```python
from build123d import *

# Parameters (mm, degrees)
SKETCH1_W           = 57.15
SKETCH1_H           = 57.15
BOSS_EXTRUDE1_DEPTH = 9.525
SKETCH5_R           = 12.281683601
SKETCH5_R_2         = 3.302
CUT_EXTRUDE1_DEPTH  = 3.175
SKETCH7_W           = 57.15
SKETCH7_H           = 57.15
CUT_EXTRUDE2_DEPTH  = 9.652
SKETCH10_R          = 3.175
CUT_EXTRUDE4_DEPTH  = 79.640756641


with BuildPart() as part:
    # Sketch1 → Boss-Extrude1 (new body)
    with BuildSketch(Plane(origin=(0, 0, 0), x_dir=(1, 0, 0), z_dir=(0, 1, 0))):
        with Locations((28.575, -28.575)):
            Rectangle(SKETCH1_W, SKETCH1_H)
    extrude(amount=BOSS_EXTRUDE1_DEPTH)

    # Sketch5 → Cut-Extrude1 (cut)
    # profile 1 of 5: a face of its own
    with BuildSketch(Plane(origin=(0, 9.525, 0), x_dir=(1, 0, 0), z_dir=(0, 1, 0))):
        with BuildLine():
            ThreePointArc((32.232759975, -45.931274041), (32.269707879, -38.244901062), (36.493054182, -31.822670864))
            ThreePointArc((36.493054182, -31.822670864), (28.575, -34.715841801), (20.656945818, -31.822670864))
            ThreePointArc((20.656945818, -31.822670864), (24.880292121, -38.244901062), (24.917240025, -45.931274041))
            ThreePointArc((24.917240025, -45.931274041), (28.575, -50.807525402), (32.232759975, -45.931274041))
        make_face()
    # profile 2 of 5: a face of its own
    with BuildSketch(Plane(origin=(0, 9.525, 0), x_dir=(1, 0, 0), z_dir=(0, 1, 0))):
        with Locations((28.575, -22.434158199)):
            Circle(SKETCH5_R)
        with Locations((28.575, -22.434158199)):
            Circle(SKETCH5_R_2, mode=Mode.SUBTRACT)
    # profile 3 of 5: a face of its own
    with BuildSketch(Plane(origin=(0, 9.525, 0), x_dir=(1, 0, 0), z_dir=(0, 1, 0))):
        with Locations((28.575, -22.434158199)):
            Circle(SKETCH5_R_2)
    # profile 4 of 5: a face of its own
    with BuildSketch(Plane(origin=(0, 9.525, 0), x_dir=(1, 0, 0), z_dir=(0, 1, 0))):
        with BuildLine():
            ThreePointArc((16.485282438, -24.597137937), (17.93875, -16.293316399), (24.403336619, -10.882665797))
            ThreePointArc((24.403336619, -10.882665797), (16.729848967, -11.329075886), (10.054780753, -7.517887219))
            ThreePointArc((10.054780753, -7.517887219), (4.002943212, -8.247474598), (6.397020778, -13.853313338))
            ThreePointArc((6.397020778, -13.853313338), (13.035141089, -17.72849765), (16.485282438, -24.597137937))
        make_face()
    # profile 5 of 5: a face of its own
    with BuildSketch(Plane(origin=(0, 9.525, 0), x_dir=(1, 0, 0), z_dir=(0, 1, 0))):
        with BuildLine():
            ThreePointArc((32.746663381, -10.882665797), (38.626736214, -15.377080109), (40.856683601, -22.434158199))
            ThreePointArc((40.856683601, -22.434158199), (40.808597958, -23.519898995), (40.664717562, -24.597137937))
            ThreePointArc((40.664717562, -24.597137937), (44.114858911, -17.72849765), (50.752979222, -13.853313338))
            ThreePointArc((50.752979222, -13.853313338), (53.147056788, -8.247474598), (47.095219247, -7.517887219))
            ThreePointArc((47.095219247, -7.517887219), (40.420151033, -11.329075886), (32.746663381, -10.882665797))
        make_face()
    extrude(amount=-CUT_EXTRUDE1_DEPTH, mode=Mode.SUBTRACT)

    # Sketch7 → Cut-Extrude2 (cut)
    with BuildSketch(Plane(origin=(0, 9.525, 0), x_dir=(1, 0, 0), z_dir=(0, 1, 0))):
        with Locations((28.575, -28.575)):
            Rectangle(SKETCH7_W, SKETCH7_H)
        with BuildLine():
            ThreePointArc((12.348348048, -5.322397737), (1.253312555, -6.659974598), (5.64245476, -16.937345621))
            ThreePointArc((5.64245476, -16.937345621), (10.720573118, -19.901836121), (13.359908547, -25.156300743))
            ThreePointArc((13.359908547, -25.156300743), (15.189119343, -30.1625), (18.610009678, -34.249742647))
            ThreePointArc((18.610009678, -34.249742647), (21.840841809, -39.162706489), (21.869106713, -45.042731239))
            ThreePointArc((21.869106713, -45.042731239), (28.575, -53.982525402), (35.280893287, -45.042731239))
            ThreePointArc((35.280893287, -45.042731239), (35.309158191, -39.162706489), (38.539990322, -34.249742647))
            ThreePointArc((38.539990322, -34.249742647), (41.960880657, -30.1625), (43.790091453, -25.156300743))
            ThreePointArc((43.790091453, -25.156300743), (46.429426882, -19.901836121), (51.50754524, -16.937345621))
            ThreePointArc((51.50754524, -16.937345621), (55.896687445, -6.659974598), (44.801651952, -5.322397737))
            ThreePointArc((44.801651952, -5.322397737), (39.695268692, -8.237931989), (33.825101131, -7.896431208))
            ThreePointArc((33.825101131, -7.896431208), (28.575, -6.977474598), (23.324898869, -7.896431208))
            ThreePointArc((23.324898869, -7.896431208), (17.454731308, -8.237931989), (12.348348048, -5.322397737))
        make_face(mode=Mode.SUBTRACT)
    extrude(amount=-CUT_EXTRUDE2_DEPTH, mode=Mode.SUBTRACT)

    # Sketch10 → Cut-Extrude4 (cut, through all)
    with BuildSketch(Plane(origin=(0, 6.35, 0), x_dir=(1, 0, 0), z_dir=(0, 1, 0))):
        with Locations(Location((28.575, -22.434158199, 0), (0, 0, 270))):
            Circle(SKETCH10_R)
    extrude(amount=-CUT_EXTRUDE4_DEPTH, mode=Mode.SUBTRACT)


solid = part.part
```
The listing builds one solid part. Answer for the finished solid, in the listing's coordinates (mm). A direction names the side the tool comes from. Give positions to 0.01 mm unless a question says otherwise; leave off trailing zeros. Write each loop counter-clockwise with the first axis right and the second up, starting at its lowest first coordinate (ties: lowest second). Pieces come first, ordered by that corner, then holes. Notation, with made-up numbers: (77.25, 0.5) - (81.25, 0.5) arc R8 cw to (81.25, 14.5) - close; hole circle Ø7 at (-29.5, -11.75). An arc over 180 degrees is marked (long way). Use one line per item in the form item = value. Start each with the question number.
1) Find section C-C on y = 7.75. Determine the outline of the cut face in (x, z) (1 decimal).
2) Consider line 1 along X through (y, z) = (9, 42.5); line 2 along Y through (x, z) = (19, 14); line 3 along Z through (x, y) = (50, 6.5). Determine where each line is inside the solid, lowest interval first. Write a range as from..to.
3) Find section B-B on z = 43. Determine the outline of the cut face in (x, y) (3 decimals), plus the area to 3 significant figures.
4) The mould has two halves that part along Z. Classify faces 3 (the face through (39.776, 4.829, 8.219)), 4 (the face through (17.909, 7.96, 28.523)), 5 (the face through (15.152, 4.829, 30.097)): pulls with the +Z half, pulls with the -Z half, needs draft (parallel to the pull), parting line crosses it, or undercut.
5) A tool of negligible diameter and unlimited length cuts with its end or side. For faces 1 (the face through (10.66, 4.83, 19.84)), 2 (the face through (12.96, 7.96, 17.65)), from which of +Z, -Z, +X, -X, +Y, -Y can it reach the whole face along a straight path? Write none if from no direction.
6) Find section D-D on x = 8. Determine the outline of the cut face in (y, z) (3 decimals).
7) Find section A-A on x = 30. Determine the outline of the cut face in (y, z) (3 decimals).
8) Flat-ended cylindrical pins translate along their axes: pin 1 Ø2 at (y, z) = (3.5, 24.5) entering from -X; pin 2 Ø5 at (y, z) = (7, 35.5) entering from -X; pin 3 Ø10 at (x, z) = (45.5, 28) entering from -Y; pin 4 Ø5 at (y, z) = (2, 38) entering from +X. Find the tip coordinate at first contact, or state that the pin passes through.
Geometry results:
q1.outline = (5.6, 16.9) arc R7 ccw (long way) to (12.3, 5.3) arc R10.3 cw to (23.3, 7.9) arc R15.5 ccw to (33.8, 7.9) arc R10.3 cw to (44.8, 5.3) arc R7 ccw (long way) to (51.5, 16.9) arc R10.3 cw to (43.8, 25.2) arc R15.5 ccw to (38.5, 34.2) arc R10.3 cw to (35.3, 45) arc R7 ccw (long way) to (21.9, 45) arc R10.3 cw to (18.6, 34.2) arc R15.5 ccw to (13.4, 25.2) arc R10.3 cw to start; hole (6.4, 13.9) arc R3.8 ccw (long way) to (10.1, 7.5) arc R13.5 cw to (24.4, 10.9) arc R12.3 ccw to (32.7, 10.9) arc R13.5 cw to (47.1, 7.5) arc R3.8 ccw (long way) to (50.8, 13.9) arc R13.5 cw to (40.7, 24.6) arc R12.3 ccw to (36.5, 31.8) arc R13.5 cw to (32.2, 45.9) arc R3.8 ccw (long way) to (24.9, 45.9) arc R13.5 cw to (20.7, 31.8) arc R12.3 ccw to (16.5, 24.6) arc R13.5 cw to start
q2.line_1 = 22.28..25.45, 31.7..34.87
q2.line_2 = 0..6.35
q2.line_3 = 3.17..6.35, 14.06..17.43
q3.outline = (22.247, 0) - (34.903, 0) - (34.903, 9.525) - (31.72, 9.525) - (31.72, 6.35) - (25.43, 6.35) - (25.43, 9.525) - (22.247, 9.525) - close
q3.area = 101 mm2
q4.face_3 = pulls with the -Z half
q4.face_4 = undercut
q4.face_5 = pulls with the +Z half
q5.face_1 = +Z, -X, +Y, -Y
q5.face_2 = +Y
q6.outline = (0, 3.202) - (9.525, 3.202) - (9.525, 6.407) - (6.35, 6.407) - (6.35, 14.353) - (9.525, 14.353) - (9.525, 17.831) - (0, 17.831) - close
q7.outline = (0, 7.043) - (9.525, 7.043) - (9.525, 10.235) - (6.35, 10.235) - (6.35, 19.597) - (0, 19.597) - close; (0, 25.271) - (6.35, 25.271) - (6.35, 50.531) - (9.525, 50.531) - (9.525, 53.836) - (0, 53.836) - close
q8.pin_1 = 12.92
q8.pin_2 = 17.29
q8.pin_3 = 0
q8.pin_4 = 37.29
